```python
from build123d import *

# Parameters (mm, degrees)
BOSS_EXTRUDE1_DEPTH = 2.54
CHAMFER1_SIZE       = 3.81
FILLET1_R           = 2.54


with BuildPart() as part:
    # Sketch1 → Boss-Extrude1 (new body)
    with BuildSketch(Plane.XY):
        Polygon((5.842, 0), (16.2941, 0), (16.2941, 33.782), (98.8441, 33.782), (98.8441, 0), (109.2962, 0), (109.2962, 2.794), (115.1382, 2.794), (115.1382, 33.782), (109.2962, 33.782), (109.2962, 43.307), (5.842, 43.307), (5.842, 33.782), (0, 33.782), (0, 2.794), (5.842, 2.794), align=None)
    extrude(amount=BOSS_EXTRUDE1_DEPTH)

    # Chamfer1
    chamfer1_edges = [part.edges().sort_by_distance(p)[0] for p in [
        (5.842, 43.307, 1.27),
        (109.2962, 43.307, 1.27),
    ]]
    chamfer(chamfer1_edges, length=CHAMFER1_SIZE)

    # Fillet1
    fillet1_edges = [part.edges().sort_by_distance(p)[0] for p in [
        (16.2941, 0, 1.27),
        (98.8441, 0, 1.27),
    ]]
    fillet(fillet1_edges, radius=FILLET1_R)


solid = part.part
```
Input: part model. Units: mm. Frame: model coordinates. A direction names the side the tool comes from. Round coordinates to 2 decimals unless told otherwise and drop trailing zeros. Loops run counter-clockwise (first coordinate to the right, second up) from the corner with the lowest first, then second, coordinate; pieces in that order, holes last.
1) Section query B-B on z = 1.8. Return the cut outline in (x, y).
Ans:
outline: (0, 2.79) - (5.84, 2.79) - (5.84, 0) - (13.75, 0) arc R2.54 ccw to (16.29, 2.54) - (16.29, 33.78) - (98.84, 33.78) - (98.84, 2.54) arc R2.54 ccw to (101.38, 0) - (109.3, 0) - (109.3, 2.79) - (115.14, 2.79) - (115.14, 33.78) - (109.3, 33.78) - (109.3, 39.5) - (105.49, 43.31) - (9.65, 43.31) - (5.84, 39.5) - (5.84, 33.78) - (0, 33.78) - close
2) Pin query (flat end, axial travel): pin 1 (0.8 mm diameter, centred on y = 35, z = 1.5, fed in from +X); pin 2 (1.3 mm diameter, centred on x = 111, z = 1.5, fed in from +Y); pin 3 (1.5 mm diameter, centred on x = 93, z = 1.5, fed in from -Y). Return the tip coordinate at first contact, or that it passes through.
Ans:
pin 1: stops at x = 109.3
pin 2: stops at y = 33.78
pin 3: stops at y = 33.78
3) Section query A-A on y = 4.5. Return the cut outline in (x, z).
Ans:
outline: (0, 0) - (16.29, 0) - (16.29, 2.54) - (0, 2.54) - close; (98.84, 0) - (115.14, 0) - (115.14, 2.54) - (98.84, 2.54) - close
4) Section query D-D on x = 68.5. Return the cut outline in (y, z).
Ans:
outline: (33.78, 0) - (43.31, 0) - (43.31, 2.54) - (33.78, 2.54) - close
5) Section query C-C on y = 37. Return the cut outline in (x, z).
Ans:
outline: (5.84, 0) - (109.3, 0) - (109.3, 2.54) - (5.84, 2.54) - close
6) Material intervals for line 1 (X direction, y = 29, z = 1.75); line 2 (Y direction, x = 50, z = 2); line 3 (X direction, y = 2, z = 1.95), sorted ascending.
Ans:
line 1: x = 0 to 16.29, 98.84 to 115.14
line 2: y = 33.78 to 43.31
line 3: x = 5.84 to 16.24, 98.9 to 109.3
7) Set-up query: faces 1 (the flat face through (57, 33.782, 1)), 2 (the flat face through (5.842, 37, 1)), 3 (the flat face through (112, 33.782, 1)). Return all of +Z, -Z, +X, -X, +Y, -Y with unobstructed straight access to the full face (end or side cutting, diameter ignored); none if empty.
Ans:
face 1: +Z, -Z, -Y
face 2: +Z, -Z, -X, +Y
face 3: +Z, -Z, +X, +Y
